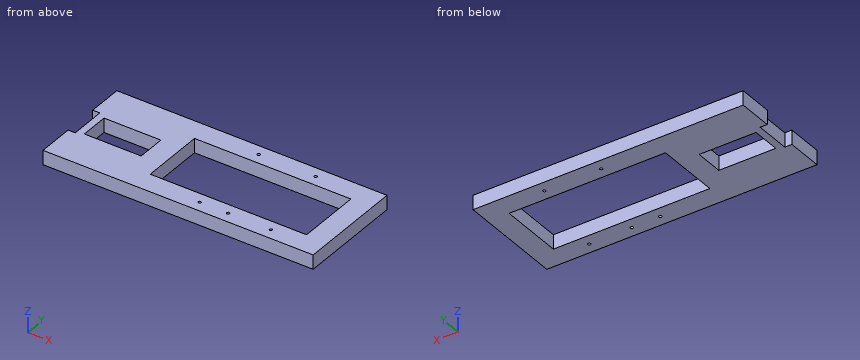
Autodesk Fusion 360 part; units mm, degrees
sketch "Sketch1" plane through (0, 0, 0) normal (0, 0, 1) x (1, 0, 0)
  line L0 (95, 37.5) -> (-95, 37.5)
  line L1 (-95, 37.5) -> (-95, -37.5)
  line L2 (-95, -37.5) -> (95, -37.5)
  line L3 (95, -37.5) -> (95, 37.5)
  line L4 (95, 37.5) -> (-95, -37.5) construction
  line L5 (-95, 37.5) -> (95, -37.5) construction
  line L6 (-45, 10) -> (-85, 10)
  line L7 (-85, 10) -> (-85, -10)
  line L8 (-85, -10) -> (-45, -10)
  line L9 (-45, -10) -> (-45, 10)
  line L10 (-45, 10) -> (-85, -10) construction
  line L11 (-85, 10) -> (-45, -10) construction
  line L12 (80, 22.5) -> (-30, 22.5)
  line L13 (-30, 22.5) -> (-30, -22.5)
  line L14 (-30, -22.5) -> (80, -22.5)
  line L15 (80, -22.5) -> (80, 22.5)
  line L16 (80, 22.5) -> (-30, -22.5) construction
  line L17 (-30, 22.5) -> (80, -22.5) construction
  line L18 (-90, 13) -> (-106.6701, 13)
  line L19 (-106.6701, 13) -> (-106.6701, -12)
  line L20 (-106.6701, -12) -> (-90, -12)
  line L21 (-90, -12) -> (-90, 13)
  point P0 (-65, 0)
  point P1 (25, 0)
  dimension "d1" = 190
  dimension "d2" = 75
  dimension "d3" = 40
  dimension "d4" = 20
  dimension "d5" = 110
  dimension "d6" = 45
  dimension "d16" = 25
extrude "Extrude1" add sketch "Sketch1" along normal blind 10 contours L0 L1 L2 L3 L18 L20 L21 | L1 L18 L20 L21
sketch "Sketch2" plane through (0, 0, 10) normal (0, 0, 1) x (-1, 0, 0)
  line L0 (-80, -22.5) -> (-80, 22.5)
  line L1 (-80, 22.5) -> (30, 22.5)
  line L2 (30, 22.5) -> (30, -22.5)
  line L3 (30, -22.5) -> (-80, -22.5)
  line L4 (45, -10) -> (45, 10)
  line L5 (45, 10) -> (85, 10)
  line L6 (85, 10) -> (85, -10)
  line L7 (85, -10) -> (45, -10)
  line L8 (-95, 37.5) -> (-95, -37.5)
  line L9 (-95, -37.5) -> (95, -37.5)
  line L10 (95, -37.5) -> (95, 37.5)
  line L11 (95, 37.5) -> (-95, 37.5)
  circle A0 centre (-10, -30) radius 1
  circle A1 centre (-50, -30) radius 1
  circle A2 centre (-10, 30) radius 1
  circle A3 centre (-30, 30) radius 1
  circle A4 centre (-60, 30) radius 1
  dimension "d9" = 2
  dimension "d10" = 2
  dimension "d11" = 2
  dimension "d12" = 2
  dimension "d13" = 2
extrude "Extrude2" cut sketch "Sketch2" against normal blind 30 contours A0 | A1 | A2 | A3 | A4
extrude "Extrude3" cut sketch "Sketch1" along normal blind 40 contours L1 L18 L20 L21 | L1 L18 L19 L20
Design review of the part built by this model. Coordinates are the model's own, in mm. Coordinates: 2 decimals unless noted, no trailing zeros. Write each loop counter-clockwise with the first axis right and the second up, starting at its lowest first coordinate (ties: lowest second). Pieces come first, ordered by that corner, then holes. Notation, with made-up numbers: (42, 27.5) - (97, 27.5) arc R25 cw to (97, 61.5) - close; hole circle Ø2 at (28.25, 17). An arc over 180 degrees is marked (long way). Use one line per item in the form item = value.
Q1. Consider section A-A (x = -70.5). Write out the cut boundary in (y, z).
Taken from the geometry:
outline = (-37.5, 0) - (-10, 0) - (-10, 10) - (-37.5, 10) - close; (10, 0) - (37.5, 0) - (37.5, 10) - (10, 10) - close
Q2. Insertion check: pin 1 Ø1.6 at (x, y) = (30, -30) entering from -Z; pin 2 Ø3 at (y, z) = (3.5, 5) entering from -X. Each pin has a flat end and moves straight along its axis. Give the tip position at first contact, or say it passes through.
Taken from the geometry:
pin_1 = through
pin_2 = -90
Q3. Consider section D-D (z = 3.5). Write out the cut boundary in (x, y), plus the area to 3 significant figures.
Taken from the geometry:
outline = (-95, -37.5) - (95, -37.5) - (95, 37.5) - (-95, 37.5) - (-95, 13) - (-90, 13) - (-90, -12) - (-95, -12) - close; hole (-85, -10) - (-45, -10) - (-45, 10) - (-85, 10) - close; hole (-30, -22.5) - (80, -22.5) - (80, 22.5) - (-30, 22.5) - close; hole circle Ø2 at (10, -30); hole circle Ø2 at (10, 30); hole circle Ø2 at (30, -30); hole circle Ø2 at (50, 30); hole circle Ø2 at (60, -30)
area = 8,360 mm^2
Q4. For probe 1 along X at (y, z) = (-2, 6); probe 2 along Y at (x, z) = (30, 5.75); probe 3 along X at (y, z) = (-30, 3), list the stretches that pass through material, from the lowest coordinate up.
Taken from the geometry:
probe_1 = -90 to -85, -45 to -30, 80 to 95
probe_2 = -37.5 to -31, -29 to -22.5, 22.5 to 37.5
probe_3 = -95 to 9, 11 to 29, 31 to 59, 61 to 95
Q5. Consider section C-C (y = 0.5). Write out the cut boundary in (x, z).
Taken from the geometry:
outline = (-90, 0) - (-85, 0) - (-85, 10) - (-90, 10) - close; (-45, 0) - (-30, 0) - (-30, 10) - (-45, 10) - close; (80, 0) - (95, 0) - (95, 10) - (80, 10) - close
Q6. Consider section B-B (y = -15.5). Write out the cut boundary in (x, z).
Taken from the geometry:
outline = (-95, 0) - (-30, 0) - (-30, 10) - (-95, 10) - close; (80, 0) - (95, 0) - (95, 10) - (80, 10) - close
